Geometry check sheet. Reference: the model listing, model coordinates, mm. Round coordinates to 2 decimals unless told otherwise and drop trailing zeros. Write each loop counter-clockwise with the first axis right and the second up, starting at its lowest first coordinate (ties: lowest second). Pieces come first, ordered by that corner, then holes.
from build123d import *

# Parameters (mm, degrees)
SKETCH1_W           = 28
SKETCH1_H           = 17
SKETCH1_W_2         = 2.55
SKETCH1_H_2         = 2.55
BOSS_EXTRUDE2_DEPTH = 1.6
SKETCH1_4_W         = 2.55
SKETCH1_4_H         = 2.55
SKETCH1_4_R         = 0.65
BOSS_EXTRUDE3_DEPTH = 1.62


with BuildPart() as part:
    # Sketch1 → Boss-Extrude2 (new body)
    with BuildSketch(Plane(origin=(0, 0, 0), x_dir=(1, 0, 0), z_dir=(0, 1, 0))):
        with Locations((126.930429576, 228.501666699)):
            Rectangle(SKETCH1_W, SKETCH1_H)
        with Locations((137.655429576, 235.376666699)):
            Rectangle(SKETCH1_W_2, SKETCH1_H_2, mode=Mode.SUBTRACT)
        with Locations((114.740971772, 235.375518488)):
            Rectangle(SKETCH1_W_2, SKETCH1_H_2, mode=Mode.SUBTRACT)
        with Locations((137.659563776, 232.245059936)):
            Rectangle(SKETCH1_W_2, SKETCH1_H_2, mode=Mode.SUBTRACT)
        with Locations((137.658202973, 225.175578697)):
            Rectangle(SKETCH1_W_2, SKETCH1_H_2, mode=Mode.SUBTRACT)
        with Locations((137.654571072, 221.735710918)):
            Rectangle(SKETCH1_W_2, SKETCH1_H_2, mode=Mode.SUBTRACT)
        with Locations((114.760575643, 221.691567702)):
            Rectangle(SKETCH1_W_2, SKETCH1_H_2, mode=Mode.SUBTRACT)
    extrude(amount=BOSS_EXTRUDE2_DEPTH)

    # Sketch1_4 → Boss-Extrude3 (add)
    with BuildSketch(Plane(origin=(0, 0, 0), x_dir=(1, 0, 0), z_dir=(0, 1, 0))):
        with Locations((137.658202973, 225.175578697)):
            Rectangle(SKETCH1_4_W, SKETCH1_4_H)
        with Locations((137.658202973, 225.175578697)):
            Circle(SKETCH1_4_R, mode=Mode.SUBTRACT)
        with Locations((137.659563776, 232.245059936)):
            Rectangle(SKETCH1_4_W, SKETCH1_4_H)
        with Locations((137.659563776, 232.245059936)):
            Circle(SKETCH1_4_R, mode=Mode.SUBTRACT)
        with Locations((137.655429576, 235.376666699)):
            Rectangle(SKETCH1_4_W, SKETCH1_4_H)
        with Locations((137.655429576, 235.376666699)):
            Circle(SKETCH1_4_R, mode=Mode.SUBTRACT)
        with Locations((114.740971772, 235.375518488)):
            Rectangle(SKETCH1_4_W, SKETCH1_4_H)
        with Locations((114.740971772, 235.384673509)):
            Circle(SKETCH1_4_R, mode=Mode.SUBTRACT)
        with Locations((114.760575643, 221.691567702)):
            Rectangle(SKETCH1_4_W, SKETCH1_4_H)
        with Locations((114.760575643, 221.691567702)):
            Circle(SKETCH1_4_R, mode=Mode.SUBTRACT)
        with Locations((137.654571072, 221.735710918)):
            Rectangle(SKETCH1_4_W, SKETCH1_4_H)
        with Locations((137.654571072, 221.735710918)):
            Circle(SKETCH1_4_R, mode=Mode.SUBTRACT)
    extrude(amount=BOSS_EXTRUDE3_DEPTH)


solid = part.part
1. Depth check by flat-ended pin: pin 1 Ø1.7 at (x, z) = (114.76, -221.69) entering from +Y. Enter the tip coordinate at first touch or a pass-through.
2. Section check B-B (z = -235.75). State how many separate pieces and enclosed holes the cut face has, plus the area to 3 significant figures.
3. Scan lines: line 1 along X through (y, z) = (1.35, -221.75); line 2 along X through (y, z) = (0.75, -235); line 3 along Z through (x, y) = (137.5, 0.55). Record each from-to range of solid material in increasing order.
4. Section check A-A (y = 0.7). Record the cut outline in (x, z).
5. Release check for a two-part mould opening along Z. For faces 1 (the face through (137.144, 0.799, -231.85)), 2 (the face through (127, 1, -220.002)), 3 (the face through (127, 0, -229)) record: +Z half, -Z half, draft (parallel to the pull), parting line (faces both ways), or undercut.
Results below:
1. pin 1: stops at y = 1.62
2. separate pieces: 3
2. enclosed holes: 0
2. area: 41.4 mm2
3. line 1: x = 112.93 to 114.11, 115.41 to 137, 138.3 to 140.93
3. line 2: x = 112.93 to 114.22, 115.26 to 137.13, 138.19 to 140.93
3. line 3: z = -237 to -236.01, -234.75 to -232.88, -231.61 to -225.81, -224.55 to -222.37, -221.1 to -220
4. outline: (112.93, -237) - (140.93, -237) - (140.93, -220) - (112.93, -220) - close; hole circle Ø1.3 at (114.74, -235.38); hole circle Ø1.3 at (114.76, -221.69); hole circle Ø1.3 at (137.65, -221.74); hole circle Ø1.3 at (137.66, -235.38); hole circle Ø1.3 at (137.66, -232.25); hole circle Ø1.3 at (137.66, -225.18)
5. face 1: undercut
5. face 2: +Z half
5. face 3: draft
